from build123d import *

# Parameters (mm, degrees)
F1_DEPTH = 19.05
F3_DEPTH = 12.7
F4_R     = 5.08
F5_W     = 5.08
F5_H     = 5.08
F6_DEPTH = 7.62


# Not quite as in the source:
# - a feature names something its author has since deleted; it is built from what else it names


with BuildPart() as f1:
    # F0 (on Top) → F1 (new body)
    with BuildSketch(Plane.XY):
        with BuildLine():
            ThreePointArc((-31.6769881083, 69.2702680826), (-41.4338257439, 40.3089202009), (-31.6769881083, 11.3475723192))
            Line((-31.6769881083, 11.3475723192), (3.9428002201, 20.5794945359))
            ThreePointArc((3.9428002201, 20.5794945359), (1.8207183061, 38.3838132659), (5.8883237652, 55.8466762304))
            Line((5.8883237652, 55.8466762304), (-31.6769881083, 69.2702680826))
        make_face()
        with BuildLine():
            ThreePointArc((-36.8869205419, 98.4383374453), (-30.0684968554, 84.6069006975), (-31.6769881083, 69.2702680826))
            Line((-31.6769881083, 69.2702680826), (5.8883237652, 55.8466762304))
            ThreePointArc((5.8883237652, 55.8466762304), (17.3296867389, 83.976336418), (11.5213459358, 113.7831434608))
            Line((11.5213459358, 113.7831434608), (-36.8869205419, 98.4383374453))
        make_face()
        with BuildLine():
            ThreePointArc((-31.6769881083, 11.3475723192), (-29.3116483225, 0.4750905822), (-34.9744334817, -9.1029340401))
            Line((-34.9744334817, -9.1029340401), (6.2283230945, -27.6920832694))
            ThreePointArc((6.2283230945, -27.6920832694), (13.878530495, -3.1399721265), (3.9428002201, 20.5794945359))
            Line((3.9428002201, 20.5794945359), (-31.6769881083, 11.3475723192))
        make_face()
        with BuildLine():
            Line((6.2283230945, -27.6920832694), (-34.9744334817, -9.1029340401))
            ThreePointArc((-34.9744334817, -9.1029340401), (-23.6676298082, -38.9988869429), (6.2283230945, -27.6920832694))
        make_face()
        with BuildLine():
            ThreePointArc((11.5213459358, 113.7831434608), (-19.9807860054, 129.1337402603), (-36.8869205419, 98.4383374453))
            Line((-36.8869205419, 98.4383374453), (11.5213459358, 113.7831434608))
        make_face()
    extrude(amount=F1_DEPTH)

    # F2 (on face) → F3 (join)
    with BuildSketch(Plane.XY.offset(19.05)):
        with BuildLine():
            ThreePointArc((-18.0934686214, 34.295540303), (-16.8286909738, 9.5468310574), (-23.8906592131, -14.2066292465))
            Line((-23.8906592131, -14.2066292465), (-6.6029457375, -22.1301615238))
            ThreePointArc((-6.6029457375, -22.1301615238), (-0.4607343944, 4.7449741554), (0, 32.3092155159))
            Line((0, 32.3092155159), (-18.0934686214, 34.295540303))
        make_face()
        with BuildLine():
            ThreePointArc((-18.0934686214, 80.9150189161), (-23.162661248, 57.6052796096), (-18.0934686214, 34.295540303))
            Line((-18.0934686214, 34.295540303), (0, 32.3092155159))
            ThreePointArc((0, 32.3092155159), (-6.5501688565, 57.2618860751), (0, 82.2145566344))
            ThreePointArc((0, 82.2145566344), (-1.439849547, 100.9781554163), (-6.6029457375, 119.0747916698))
            Line((-6.6029457375, 119.0747916698), (-24.2383088917, 112.1475473046))
            ThreePointArc((-24.2383088917, 112.1475473046), (-19.2665441206, 96.9049694563), (-18.0934686214, 80.9150189161))
        make_face()
    extrude(amount=F3_DEPTH)

    # F4
    f4_edges = [f1.edges().sort_by_distance(p)[0] for p in [
        (-23.890659, -14.206629, 25.4),
        (-6.602946, -22.130162, 25.4),
        (-6.602946, 119.074792, 25.4),
        (-24.238309, 112.147547, 25.4),
        (0, 82.214557, 25.4),
        (0, 32.309216, 25.4),
        (-18.093469, 80.915019, 25.4),
        (-18.093469, 34.29554, 25.4),
    ]]
    fillet(f4_edges, radius=F4_R)

    # F5 (on Top) → F6 (join)
    with BuildSketch(Plane.XY):
        with Locations((-26.6524679592, -24.0524802357)):
            Rectangle(F5_W, F5_H)
        with Locations((-0.8571739626, -22.7268876201)):
            Rectangle(F5_W, F5_H)
        with Locations((-27.3225028068, -5.8132838458)):
            Rectangle(F5_W, F5_H)
        with Locations((-5.4335221648, -10.0806634873)):
            Rectangle(F5_W, F5_H)
        with Locations((-26.5202838928, 9.5173716545)):
            Rectangle(F5_W, F5_H)
        with Locations((-7.7564124949, 14.4977606833)):
            Rectangle(F5_W, F5_H)
        with Locations((-32.2857946157, 33.5665121675)):
            Rectangle(F5_W, F5_H)
        with Locations((-10.6263644993, 33.2580432296)):
            Rectangle(F5_W, F5_H)
        with Locations((-31.4632356167, 49.4136251509)):
            Rectangle(F5_W, F5_H)
        with Locations((-9.5391534269, 49.3687652051)):
            Rectangle(F5_W, F5_H)
        with Locations((-27.4613853544, 70.2730193734)):
            Rectangle(F5_W, F5_H)
        with Locations((-7.6474579982, 71.8173533678)):
            Rectangle(F5_W, F5_H)
        with Locations((-27.4252351373, 89.291498065)):
            Rectangle(F5_W, F5_H)
        with Locations((-5.7547562756, 94.7942361236)):
            Rectangle(F5_W, F5_H)
        with Locations((-29.7734234482, 104.6168133616)):
            Rectangle(F5_W, F5_H)
        with Locations((-7.6474579982, 106.1389820957)):
            Rectangle(F5_W, F5_H)
    extrude(amount=-F6_DEPTH)


solid = f1.part
Verification items for the finished model (mm, model axes). A direction names the side the tool comes from. Give positions to 0.01 mm unless a question says otherwise; leave off trailing zeros. Order: outer loops, then holes, each group sorted by start corner. A loop starts at its lowest first (then second) coordinate and runs counter-clockwise, first axis right, second up. Notation, with made-up numbers: M -18.75,23 L 35.25,23 A27 ccw 35.25,49 Z; hole C 43,8.25 d6. An arc over 180 degrees is marked long. Answer as a JSON object with one key per item and string values. Group by question number.
1) Access from +Z, -Z, +X, -X, +Y, -Y to the whole of each face (thin tool, end or side, straight path). Record for faces 1 (the face through (-27, 72.813, -4)), 2 (the face through (-5.107, 106, -4)), 3 (the face through (-8, 108.679, -4)).
2) Cross-section at C-C (y = 40.5). Enter the section's corners in (x, z), then the cut area to 3 significant figures.
3) Cross-section at B-B (y = 14). Enter the section's corners in (x, z).
4) Cross-section at A-A (z = 8.5). Enter the section's corners in (x, y).
5) Scan lines: line 1 along Y through (x, z) = (-30.5, -2); line 2 along Y through (x, z) = (-32, 4.5); line 3 along Y through (x, z) = (0, -5.5). Record each from-to range of solid material in increasing order. Write a range as [from, to].
6) Depth check by flat-ended pin: pin 1 Ø2.5 at (y, z) = (71, -2.5) entering from +X; pin 2 Ø2 at (x, z) = (-13, -3.5) entering from +Y; pin 3 Ø1.5 at (y, z) = (89, -3.5) entering from +X. Enter the tip coordinate at first touch or a pass-through.
7) Mould release check, pull along X, two halves, no side actions. Record for faces 4 (the face through (-11, 50, 31.75)), 5 (the face through (-19.463, 129.292, 9.392)), 6 (the face through (-10.187, 72, -4)): released by +X, released by -X, zero draft, split by the parting line, or undercut.
Result sheet:
{
 "1": {"face 1": "-Z, -X", "face 2": "-Z, +X, +Y", "face 3": "-Z, +X, -X, +Y"},
 "2": {"outline": "M -41.43,0 L 1.98,0 L 1.98,19.05 L -3.71,19.05 L -3.71,31.75 L -20.49,31.75 L -20.49,19.05 L -41.43,19.05 Z", "area": "1,040 mm2"},
 "3": {"outline": "M -33.55,0 L -10.3,0 L -10.3,-7.62 L -5.22,-7.62 L -5.22,0 L 8.81,0 L 8.81,19.05 L 0.33,19.05 L 0.33,31.75 L -16.43,31.75 L -16.43,19.05 L -33.55,19.05 Z"},
 "4": {"outline": "M -36.89,98.44 A27.78 cw -31.68,69.27 A47.86 ccw -31.68,11.35 A15.22 cw -34.97,-9.1 A22.6 ccw 6.23,-27.69 A37.56 ccw 3.94,20.58 A51.86 cw 5.89,55.85 A53.21 ccw 11.52,113.78 A25.42 ccw Z"},
 "5": {"line 1": "y = [31.03, 36.11], [46.87, 51.95], [102.08, 107.16]", "line 2": "y = [-32.54, -6.02], [11.78, 68.84], [90.94, 120.97]", "line 3": "y = [-25.27, -20.19]"},
 "6": {"pin 1": "stops at x = -5.11", "pin 2": "stops at y = 51.91", "pin 3": "stops at x = -24.89"},
 "7": {"face 4": "zero draft", "face 5": "split by the parting line", "face 6": "undercut"}
}
